Read the model definition and answer for the solid it produces. Units are mm, in the model's axes. A direction names the side the tool comes from. Coordinates: 2 decimals unless noted, no trailing zeros. Write each loop counter-clockwise with the first axis right and the second up, starting at its lowest first coordinate (ties: lowest second). Pieces come first, ordered by that corner, then holes. Notation, with made-up numbers: M 21.25,-20.75 L 55.25,-20.75 A27 ccw 55.25,11.25 Z; hole C 52.5,-8 d10. An arc over 180 degrees is marked long. Use a Markdown table: item, result. Add a question column.
Autodesk Inventor part; units mm, degrees
ref_plane "YZ Plane" through (0, 0, 0) normal (1, 0, 0) x (0, 1, 0)
ref_plane "XZ Plane" through (0, 0, 0) normal (0, 1, 0) x (-1, 0, 0)
ref_plane "XY Plane" through (0, 0, 0) normal (0, 0, 1) x (1, 0, 0)
sketch "Skizze3" plane through (0, 0, 0) normal (0, 0, 1) x (1, 0, 0)
  line L0 (0, 0) -> (-10, 0)
  line L1 (-10, 0) -> (-10, -25)
  line L2 (-10, -25) -> (0, -25)
  line L3 (0, -25) -> (0, 0)
  dimension "d4" = 10
  dimension "d5" = 25
extrude "Extrusion3" add sketch "Skizze3" along normal blind 6
sketch "Skizze4" plane through (-10, -25, 0) normal (0, -1, 0) x (1, 0, 0)
  line L0 (10, 0) -> (10, 6)
  line L1 (0, 0) -> (0, 6)
  point P0 (6, 3)
  point P1 (0, 3)
  dimension "d8" = 4
hole "Bohrung1" at (-4, -25, 3) direction (0, 1, 0) diameter 3 depth 10 tip angle 118
thread "Gewinde1"
sketch "Skizze5" plane through (0, -25, 0) normal (1, 0, 0) x (0, 0, -1)
  line L0 (0, 25) -> (-6, 25)
  line L1 (0, 0) -> (-6, 0)
  point P0 (-3, 17)
  point P1 (-3, 25)
  dimension "d18" = 17
hole "Bohrung2" at (0, -8, 3) direction (-1, 0, 0) diameter 3 depth 8 tip angle 118
thread "Gewinde2"
fillet "Rundung1" radius 2 1 edges at (-10, 0, 3)
properties part number "getriebe_winkel" material "Acryl"
Item 1: Consider probe 1 along Z at (x, y) = (-5.5, -8); probe 2 along Y at (x, z) = (-2, 3); probe 3 along X at (y, z) = (-18.25, 3). Determine where each line is inside the solid, lowest interval first.
Item 2: Find section B-B on x = -7. Give the vertices of the cut face in (y, z), then the cut area to 3 significant figures.
Item 3: Find section A-A on y = -16.5. Give the vertices of the cut face in (x, z).
Item 4: For faces 1 (the flat face through (-5, -12, 6)), 2 (the cylindrical face through (-4.45, -19.93, 1.57)), 3 (the cylindrical face through (-4.06, -6.67, 2.31)), determine the directions among +Z, -Z, +X, -X, +Y, -Y from which every point of the face is accessible in a straight line to the end or side of a thin tool.
Item 5: This flat-tipped pin is pushed along its axis until it touches: pin 1 (1.8 mm diameter, centred on x = -4, z = 3, fed in from -Y). Where does it stop, or does it pass through?
Item 6: Determine the mould class of faces 4 (the flat face through (-10, -13, 3)), 5 (the flat face through (-6, -25, 3)), 6 (the conical face through (-8.745, -8.1, 2.759)), 7 (the flat face through (-4, 0, 3)) for opening direction Y: pulls with the +Y half, pulls with the -Y half, needs draft (parallel to the pull), parting line crosses it, or undercut.
Geometry says:
| question | item | result |
|---|---|---|
| 1 | probe 1 | z = 0 to 1.5, 4.5 to 6 |
| 1 | probe 2 | y = -25 to -9.5, -6.5 to 0 |
| 1 | probe 3 | x = -10 to -5.5, -2.5 to 0 |
| 2 | outline | M -25,0 L 0,0 L 0,6 L -25,6 Z; hole C -8,3 d3 |
| 2 | area | 143 mm2 |
| 3 | outline | M -10,0 L 0,0 L 0,6 L -10,6 Z; hole C -4,3 d3 |
| 4 | face 1 | +Z, +X, -X, +Y, -Y |
| 4 | face 2 | -Y |
| 4 | face 3 | +X |
| 5 | pin 1 | stops at y = -14.64 |
| 6 | face 4 | needs draft |
| 6 | face 5 | pulls with the -Y half |
| 6 | face 6 | undercut |
| 6 | face 7 | pulls with the +Y half |
